CAD build for the part. Positions are in the model's coordinates, mm. Face numbers are marked on the shaded views. A direction names the side the tool comes from. Give positions to 0.01 mm unless a question says otherwise; leave off trailing zeros.
from build123d import *

# Parameters (mm, degrees)
BOSS_EXTRUDE1_DEPTH = 155
CUT_EXTRUDE1_REACH  = 230.601
SKETCH2_W           = 102
SKETCH2_H           = 25
CUT_EXTRUDE2_REACH  = 281.613
SKETCH3_W           = 102
SKETCH3_H           = 25
FILLET1_R           = 5
FILLET2_R           = 10
FILLET4_R           = 10
SHELL1_T            = -2
CUT_EXTRUDE3_REACH  = 280.913
SKETCH9_W           = 92
SKETCH9_H           = 20


with BuildPart() as part:
    # Sketch1 → Boss-Extrude1 (new body)
    with BuildSketch(Plane(origin=(0, 0, 0), x_dir=(1, 0, 0), z_dir=(0, 1, 0))):
        Polygon((63.508529611, 110), (-63.508529611, 110), (-127.017059222, 0), (-63.508529611, -110), (63.508529611, -110), (127.017059222, 0), align=None)
    extrude(amount=BOSS_EXTRUDE1_DEPTH)

    # Sketch2 → Cut-Extrude1 (cut, up to next)
    with BuildSketch(Plane(origin=(0, 155, 0), x_dir=(1, 0, 0), z_dir=(0, 1, 0)), mode=Mode.PRIVATE) as cut_extrude1_sk1:
        with Locations((0, -97.5)):
            Rectangle(SKETCH2_W, SKETCH2_H)
    cut_extrude1_tool1 = extrude(cut_extrude1_sk1.sketch, amount=-CUT_EXTRUDE1_REACH, mode=Mode.PRIVATE) & part.part
    add(cut_extrude1_tool1.solids().sort_by_distance((0, 155, 97.5))[0], mode=Mode.SUBTRACT)

    # Sketch3 → Cut-Extrude2 (cut, up to next)
    with BuildSketch(Plane.XY.offset(85), mode=Mode.PRIVATE) as cut_extrude2_sk1:
        with Locations((0, 12.5)):
            Rectangle(SKETCH3_W, SKETCH3_H)
    cut_extrude2_tool1 = extrude(cut_extrude2_sk1.sketch, amount=-CUT_EXTRUDE2_REACH, mode=Mode.PRIVATE) & part.part
    add(cut_extrude2_tool1.solids().sort_by_distance((0, 12.5, 85))[0], mode=Mode.SUBTRACT)

    # Fillet1
    fillet1_edges = [part.edges().sort_by_distance(p)[0] for p in [
        (51, 90, 85),
        (-51, 90, 85),
        (-51, 25, -12.5),
        (51, 25, -12.5),
        (0, 25, 85),
    ]]
    fillet(fillet1_edges, radius=FILLET1_R)

    # Fillet2
    fillet2_edges = [part.edges().sort_by_distance(p)[0] for p in [
        (127.017059222, 77.5, 0),
        (63.508529611, 77.5, 110),
        (-63.508529611, 77.5, 110),
        (-127.017059222, 77.5, 0),
        (-63.508529611, 77.5, -110),
        (63.508529611, 77.5, -110),
    ]]
    fillet(fillet2_edges, radius=FILLET2_R)

    # Fillet4
    fillet4_edges = [part.edges().sort_by_distance(p)[0] for p in [
        (54.367513459, 0, 110),
        (-54.367513459, 0, -110),
        (95.262794416, 0, 55),
        (54.367513459, 0, -110),
        (95.262794416, 0, -55),
        (62.735026919, 0, -108.660254038),
        (125.470053838, 0, 0),
        (62.735026919, 0, 108.660254038),
        (-95.262794416, 0, -55),
        (-54.367513459, 0, 110),
        (-95.262794416, 0, 55),
        (-62.735026919, 0, 108.660254038),
        (-125.470053838, 0, 0),
        (-62.735026919, 0, -108.660254038),
    ]]
    fillet(fillet4_edges, radius=FILLET4_R)

    # Shell1
    shell1_openings = [part.faces().sort_by_distance(p)[0] for p in [
        (0, 155, -6.295757264),
    ]]
    offset(amount=SHELL1_T, openings=shell1_openings, kind=Kind.INTERSECTION)

    # Sketch9 → Cut-Extrude3 (cut, up to next)
    with BuildSketch(Plane.XY.offset(85), mode=Mode.PRIVATE) as cut_extrude3_sk1:
        with Locations((0, 145)):
            Rectangle(SKETCH9_W, SKETCH9_H)
    cut_extrude3_tool1 = extrude(cut_extrude3_sk1.sketch, amount=-CUT_EXTRUDE3_REACH, mode=Mode.PRIVATE) & part.part
    add(cut_extrude3_tool1.solids().sort_by_distance((0, 145, 85))[0], mode=Mode.SUBTRACT)


solid = part.part
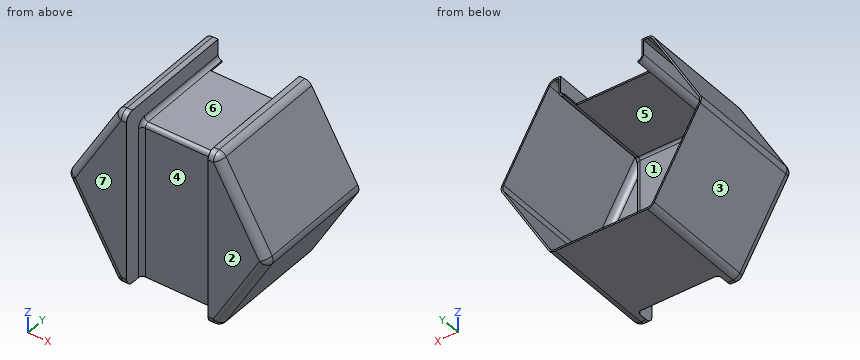
1. Mould opens along Z. For the marked faces 1, 2 and 3 say: released by +Z, released by -Z, zero draft, split by the parting line, or undercut.
2. Pin check, flat tips, straight feed: P1, Ø1, axis at y = 64, z = 11.5, coming from the -X side; P2, Ø1, axis at y = 140.5, z = 84, coming from the -X side; P3, Ø1.5, axis at y = 83, z = 8, coming from the -X side. Stop position of each tip, or through.
3. 3-axis set-ups, long thin cutter, end or side, ignore diameter. For the marked faces 4, 5, 6 and 7: which of +Z, -Z, +X, -X, +Y, -Y reach the whole face in a straight line?
4. Wall check: line 1 (Z direction, x = -67, y = 48); line 2 (Z direction, x = -10, y = 77); line 3 (X direction, y = 29.5, z = 97.5). Give the ranges that are in metal, low to high.
5. Saw through at A-A on y = 13. State how many separate pieces and enclosed holes the cut face has, plus the area to 3 significant figures.
Reported:
1. face 1: undercut
1. face 2: zero draft
1. face 3: released by -Z
2. P1: stops at x = -120.67
2. P2: stops at x = -78.81
2. P3: stops at x = -122.83
3. face 4: +Z, -Z, -Y
3. face 5: +Y
3. face 6: +Z, +Y, -Y
3. face 7: +Z, -Z, +X, -X, -Y
4. line 1: z = -103.95 to -99.95, 99.95 to 103.95
4. line 2: z = -110 to -108, 83 to 85
4. line 3: x = -70.73 to -68.42, -53 to -51, 51 to 53, 68.42 to 70.73
5. separate pieces: 2
5. enclosed holes: 2
5. area: 1,950 mm2
